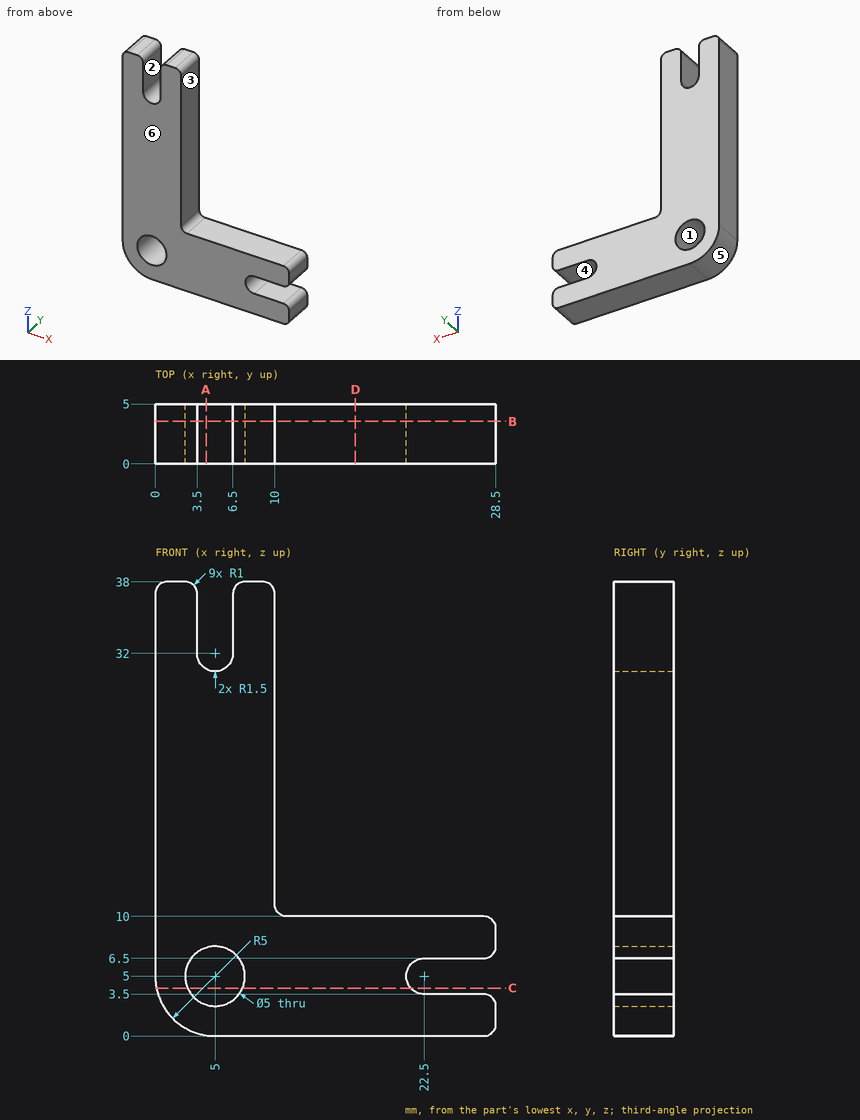
Geometry check sheet. Reference: drawing and pictorial views, mm from the part's lowest x, y, z. A direction names the side the tool comes from. Round coordinates to 2 decimals unless told otherwise and drop trailing zeros. Order: outer loops, then holes, each group sorted by start corner. A loop starts at its lowest first (then second) coordinate and runs counter-clockwise, first axis right, second up. Notation, with made-up numbers: (-19, 13) - (0, 13) arc R22 ccw to (0, 34) - close; hole circle Ø6 at (89, 44). An arc over 180 degrees is marked (long way). One line per question, with ' | ' between items. Start each with the question number.
(1) Sectioned sample at B-B on y = 3.55. Record the cut outline in (x, z), and give its area (3 significant figures).
(2) Access from +Z, -Z, +X, -X, +Y, -Y to the whole of each face (thin tool, end or side, straight path). Record for the marked faces 1, 2 and 3.
(3) Sectioned sample at C-C on z = 4. Record the cut outline in (x, y), and give its area (3 significant figures).
(4) Sectioned sample at D-D on x = 16.75. Record the cut outline in (y, z), and give its area (3 significant figures).
(5) Depth check by flat-ended pin: pin 1 Ø2.5 at (y, z) = (2.5, 19.5) entering from +X; pin 2 Ø1.5 at (x, y) = (22, 2) entering from +Z; pin 3 Ø1.5 at (x, y) = (4, 1.5) entering from -Z. Enter the tip coordinate at first touch or a pass-through.
(6) Release check for a two-part mould opening along Z. For the marked faces 4, 5 and 6 record: released by +Z, released by -Z, zero draft, split by the parting line, or undercut.
(7) Sectioned sample at A-A on x = 4.25. Record the cut outline in (y, z).
(8) Thickness scan on L1, parallel to X at y = 2.15, z = 33; L2, parallel to X at y = 2.75, z = 24. Record the ranges inside material, lowest first. Write a range as [from, to].
Conclusion:
1) outline: (0, 5) arc R5 ccw to (5, 0) - (27.5, 0) arc R1 ccw to (28.5, 1) - (28.5, 2.5) arc R1 ccw to (27.5, 3.5) - (22.5, 3.5) arc R1.5 cw to (22.5, 6.5) - (27.5, 6.5) arc R1 ccw to (28.5, 7.5) - (28.5, 9) arc R1 ccw to (27.5, 10) - (11, 10) arc R1 cw to (10, 11) - (10, 37) arc R1 ccw to (9, 38) - (7.5, 38) arc R1 ccw to (6.5, 37) - (6.5, 32) arc R1.5 cw to (3.5, 32) - (3.5, 37) arc R1 ccw to (2.5, 38) - (1, 38) arc R1 ccw to (0, 37) - close; hole circle Ø5 at (5, 5) | area: 495 mm2
2) face 1: +Y, -Y | face 2: +Z, +Y, -Y | face 3: +Z, +X, +Y, -Y
3) outline: (0.1, 0) - (2.71, 0) - (2.71, 5) - (0.1, 5) - close; (7.29, 0) - (21.38, 0) - (21.38, 5) - (7.29, 5) - close | area: 83.5 mm2
4) outline: (0, 0) - (5, 0) - (5, 10) - (0, 10) - close | area: 50.0 mm2
5) pin 1: stops at x = 10 | pin 2: stops at z = 10 | pin 3: stops at z = 0.01
6) face 4: undercut | face 5: released by -Z | face 6: zero draft
7) outline: (0, 0.06) - (5, 0.06) - (5, 2.62) - (0, 2.62) - close; (0, 7.38) - (5, 7.38) - (5, 30.7) - (0, 30.7) - close
8) L1: x = [0, 3.5], [6.5, 10] | L2: x = [0, 10]
